Verification items for the finished model (mm, model axes). Face numbers are marked on the shaded views. A direction names the side the tool comes from. Coordinates: 2 decimals unless noted, no trailing zeros. Write each loop counter-clockwise with the first axis right and the second up, starting at its lowest first coordinate (ties: lowest second). Pieces come first, ordered by that corner, then holes. Notation, with made-up numbers: (-21, 45.5) -> (6, 45.5) arc R34 cw to (6, 79.5) -> close; hole circle Ø2 at (33.5, -22.5). An arc over 180 degrees is marked (long way). Answer in a Markdown table with one row per item.
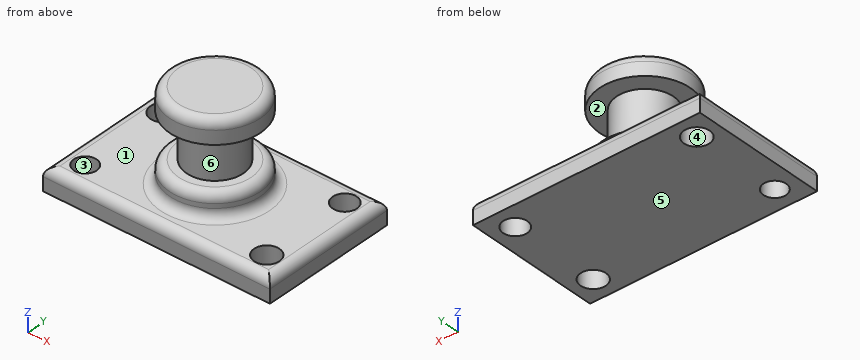
```python
from build123d import *

# Parameters (mm, degrees)
F0_W     = 127
F0_H     = 76.2
F1_DEPTH = 12.7
F2_R     = 7.198910885
F2_R_2   = 6.7607209877
F2_R_3   = 7.0919024912
F2_R_4   = 6.3659189417
F3_DEPTH = 12.701
F4_W     = 25.4
F4_H     = 50.8
F6_W     = 20.640426774
F6_H     = 25.4
F8_R     = 5.08


with BuildPart() as f1:
    # F0 (on Top) → F1 (new body)
    with BuildSketch(Plane.XY):
        Rectangle(F0_W, F0_H)
    extrude(amount=F1_DEPTH)

    # F2 (on face) → F3 (cut, through all)
    with BuildSketch(Plane.XY.offset(12.7)):
        with Locations((-50.8, 25.4)):
            Circle(F2_R)
        with Locations((50.8, 25.4)):
            Circle(F2_R_2)
        with Locations((50.8, -25.4)):
            Circle(F2_R_3)
        with Locations((-50.8, -25.4)):
            Circle(F2_R_4)
    extrude(amount=-F3_DEPTH, mode=Mode.SUBTRACT)

    # F4 (on Front) → F5 (revolve)
    with BuildSketch(Plane.XZ):
        with Locations((12.7, 38.1)):
            Rectangle(F4_W, F4_H)
    revolve(axis=Axis((0, 0, 38.1), (0, 0, 1)))

    # F6 (on Front) → F7 (revolve, cut)
    with BuildSketch(Plane.XZ):
        with Locations((26.1877048761, 38.1)):
            Rectangle(F6_W, F6_H)
    revolve(axis=Axis((0, 0, 12.7), (0, 0, 1)), mode=Mode.SUBTRACT)

    # F8
    f8_edges = [f1.edges().sort_by_distance(p)[0] for p in [
        (-25.4, 0, 63.5),
        (-25.4, 0, 12.7),
        (-25.4, 0, 25.4),
        (0, -38.1, 12.7),
        (63.5, 0, 12.7),
        (0, 38.1, 12.7),
        (-63.5, 0, 12.7),
    ]]
    fillet(f8_edges, radius=F8_R)


solid = f1.part
```
1. Sectioned sample at A-A, the plane x = -50.8. Record the cut outline in (y, z), and give its area (3 significant figures).
Findings below:
| item | result |
|---|---|
| outline | (-38.1, 0) -> (-31.77, 0) -> (-31.77, 12.7) -> (-33.02, 12.7) arc R5.08 ccw to (-38.1, 7.62) -> close; (-19.03, 0) -> (18.2, 0) -> (18.2, 12.7) -> (-19.03, 12.7) -> close; (32.6, 0) -> (38.1, 0) -> (38.1, 7.62) arc R5.08 ccw to (33.02, 12.7) -> (32.6, 12.7) -> close |
| area | 612 mm² |
2. Sectioned sample at C-C, the plane x = 0. Record the cut outline in (y, z).
Findings below:
| item | result |
|---|---|
| outline | (-38.1, 0) -> (38.1, 0) -> (38.1, 7.62) arc R5.08 ccw to (33.02, 12.7) -> (30.48, 12.7) arc R5.08 cw to (25.4, 17.78) -> (25.4, 20.32) arc R5.08 ccw to (20.32, 25.4) -> (15.87, 25.4) -> (15.87, 50.8) -> (25.4, 50.8) -> (25.4, 58.42) arc R5.08 ccw to (20.32, 63.5) -> (-20.32, 63.5) arc R5.08 ccw to (-25.4, 58.42) -> (-25.4, 50.8) -> (-15.87, 50.8) -> (-15.87, 25.4) -> (-20.32, 25.4) arc R5.08 ccw to (-25.4, 20.32) -> (-25.4, 17.78) arc R5.08 cw to (-30.48, 12.7) -> (-33.02, 12.7) arc R5.08 ccw to (-38.1, 7.62) -> close |
3. Sectioned sample at D-D, the plane z = 47. Record the cut outline in (x, y), and give its area (3 significant figures).
Findings below:
| item | result |
|---|---|
| outline | circle Ø31.73 at (0, 0) |
| area | 791 mm² |
4. Material ranges on probe 1 along X at (y, z) = (25, 3); probe 2 along Y at (x, z) = (51, 4.5); probe 3 along Y at (x, z) = (-50.8, 2.5), recorded low to high. Write a range as from..to.
Findings below:
| item | result |
|---|---|
| probe 1 | x = -63.5..-57.99, -43.61..44.05, 57.55..63.5 |
| probe 2 | y = -38.1..-32.49, -18.31..18.64, 32.16..38.1 |
| probe 3 | y = -38.1..-31.77, -19.03..18.2, 32.6..38.1 |
5. Go/stop test with flat-tipped pins: pin 1 (10 mm diameter, centred on x = 18.5, z = 40.5, fed in from +Y); pin 2 (10 mm diameter, centred on y = 17, z = 26, fed in from +X); pin 3 (1.5 mm diameter, centred on x = -5, z = 44.5, fed in from -Y); pin 4 (11 mm diameter, centred on x = 50.8, y = 25.4, fed in from -Z). Record where each tip stops, or that it passes through.
Findings below:
| item | result |
|---|---|
| pin 1 | stops at y = 8.34 |
| pin 2 | stops at x = 20.98 |
| pin 3 | stops at y = -15.29 |
| pin 4 | passes through |
6. Sectioned sample at B-B, the plane y = 0. Record the cut outline in (x, z), and give its area (3 significant figures).
Findings below:
| item | result |
|---|---|
| outline | (-63.5, 0) -> (63.5, 0) -> (63.5, 7.62) arc R5.08 ccw to (58.42, 12.7) -> (30.48, 12.7) arc R5.08 cw to (25.4, 17.78) -> (25.4, 20.32) arc R5.08 ccw to (20.32, 25.4) -> (15.87, 25.4) -> (15.87, 50.8) -> (25.4, 50.8) -> (25.4, 58.42) arc R5.08 ccw to (20.32, 63.5) -> (-20.32, 63.5) arc R5.08 ccw to (-25.4, 58.42) -> (-25.4, 50.8) -> (-15.87, 50.8) -> (-15.87, 25.4) -> (-20.32, 25.4) arc R5.08 ccw to (-25.4, 20.32) -> (-25.4, 17.78) arc R5.08 cw to (-30.48, 12.7) -> (-58.42, 12.7) arc R5.08 ccw to (-63.5, 7.62) -> close |
| area | 3,690 mm² |
7. Release check for a two-part mould opening along Z. For the marked faces 4, 5 and 6 record: released by +Z, released by -Z, zero draft, split by the parting line, or undercut.
Findings below:
| item | result |
|---|---|
| face 4 | zero draft |
| face 5 | released by -Z |
| face 6 | undercut |
8. Access from +Z, -Z, +X, -X, +Y, -Y to the whole of each face (thin tool, end or side, straight path). Record for the marked faces 1, 2 and 3.
Findings below:
| item | result |
|---|---|
| face 1 | +Z |
| face 2 | none |
| face 3 | +Z, -Z |
